Autodesk Inventor part; units mm, degrees
ref_plane "tube_front_XY" through (0, 0, 0) normal (1, 0, 0) x (0, 0, -1)
ref_plane "tube_front_YZ" through (0, 0, 0) normal (0, 0, -1) x (0, 1, 0)
ref_plane "tube_front_ZX" through (0, 0, 0) normal (0, 1, 0) x (1, 0, 0)
sketch "Sketch_1" plane through (0, 0, 0) normal (0, 0, 1) x (1, 0, 0)
  line L0 (414.3629, 0) -> (0, 0)
  arc A0 (-0.6395, 13.2842) -> (-0.6395, 13.1046) centre (-0.5497, 13.1944) ccw
  line L1 (-0.6395, 13.1046) -> (-0.381, 12.846)
  line L2 (-0.381, 12.846) -> (0, 12.846)
  line L3 (0, 12.846) -> (0.762, 13.6081)
  line L4 (0.762, 13.6081) -> (413.6009, 13.6081)
  line L5 (413.6009, 13.6081) -> (414.3629, 12.846)
  line L6 (414.3629, 12.846) -> (414.7439, 12.846)
  line L7 (414.7439, 12.846) -> (415.0024, 13.1046)
  arc A1 (415.0024, 13.1046) -> (415.0024, 13.2842) centre (414.9126, 13.1944) ccw
  line L8 (415.0024, 13.2842) -> (414.3747, 13.9119)
  arc A2 (414.3747, 13.9119) -> (413.8359, 14.1351) centre (413.8359, 13.3731) ccw
  line L9 (413.8359, 14.1351) -> (0.527, 14.1351)
  arc A3 (0.527, 14.1351) -> (-0.0118, 13.9119) centre (0.527, 13.3731) ccw
  line L10 (-0.0118, 13.9119) -> (-0.6395, 13.2842)
revolve "Revolution1" add sketch "Sketch_1" angle 360 about axis through (414.3629, 0, 0) along (1, 0, 0)
ref_plane "tube_front_XY" through (0, 0, 0) normal (1, 0, 0) x (0, 0, -1)
ref_plane "tube_front_YZ" through (0, 0, 0) normal (0, 0, -1) x (0, 1, 0)
ref_plane "tube_front_ZX" through (0, 0, 0) normal (0, 1, 0) x (1, 0, 0)
ref_plane "tube_rear_XY" through (414.3629, 0, 0) normal (1, 0, 0) x (0, 0, -1)
ref_plane "tube_rear_YZ" through (414.3629, 0, 0) normal (0, 0, -1) x (0, 1, 0)
ref_plane "tube_rear_ZX" through (414.3629, 0, 0) normal (0, 1, 0) x (1, 0, 0)
ref_plane "cp1_XY" through (207.1815, 14.1351, 0) normal (1, 0, 0) x (0, 0, -1)
ref_plane "cp1_YZ" through (207.1815, 14.1351, 0) normal (0, 0, -1) x (0, 1, 0)
ref_plane "cp1_ZX" through (207.1815, 14.1351, 0) normal (0, 1, 0) x (1, 0, 0)
ref_plane "cp2_XY" through (207.1815, 0, -14.1351) normal (1, 0, 0) x (0, 0, -1)
ref_plane "cp2_YZ" through (207.1815, 0, -14.1351) normal (0, 0, -1) x (0, 1, 0)
ref_plane "cp2_ZX" through (207.1815, 0, -14.1351) normal (0, 1, 0) x (1, 0, 0)
ref_plane "cp3_XY" through (207.1815, -14.1351, 0) normal (1, 0, 0) x (0, 0, -1)
ref_plane "cp3_YZ" through (207.1815, -14.1351, 0) normal (0, 0, -1) x (0, 1, 0)
ref_plane "cp3_ZX" through (207.1815, -14.1351, 0) normal (0, 1, 0) x (1, 0, 0)
ref_plane "cp4_XY" through (207.1815, 0, 14.1351) normal (1, 0, 0) x (0, 0, -1)
ref_plane "cp4_YZ" through (207.1815, 0, 14.1351) normal (0, 0, -1) x (0, 1, 0)
ref_plane "cp4_ZX" through (207.1815, 0, 14.1351) normal (0, 1, 0) x (1, 0, 0)
properties part number "09R-16.31350" material "Stainless Steel"
Geometry check sheet. Reference: the model listing, model coordinates, mm. Coordinates: 2 decimals unless noted, no trailing zeros. Order: outer loops, then holes, each group sorted by start corner. A loop starts at its lowest first (then second) coordinate and runs counter-clockwise, first axis right, second up.
Item 1: Scan lines: line 1 along Y through (x, z) = (321.5, -1.25); line 2 along Z through (x, y) = (-0.3, 0); line 3 along Z through (x, y) = (414.4, 0). Record each from-to range of solid material in increasing order.
Item 2: Section check A-A (y = 0). Enter the section's corners in (x, z).
Item 3: Mould release check, pull along X, two halves, no side actions. Record for faces 1 (the cylindrical face through (210.07, -10.8, -8.28)), 2 (the cylindrical face through (414.56, -2.78, -12.54)): released by +X, released by -X, zero draft, split by the parting line, or undercut.
Item 4: Section check C-C (x = 251.5). Enter the section's corners in (y, z), plus the area to 3 significant figures.
Item 5: Depth check by flat-ended pin: pin 1 (10 mm diameter, centred on y = 1, z = -7.5, fed in from +X); pin 2 (2 mm diameter, centred on x = 327, y = 10, fed in from +Z); pin 3 (3 mm diameter, centred on x = 300.5, y = 8, fed in from +Z); pin 4 (6 mm diameter, centred on x = 365.5, z = -7.5, fed in from +Y). Enter the tip coordinate at first touch or a pass-through.
Check sheet entries:
1. line 1: y = -14.08 to -13.55, 13.55 to 14.08
1. line 2: z = -13.62 to -12.85, 12.85 to 13.62
1. line 3: z = -13.89 to -12.85, 12.85 to 13.89
2. outline: (-0.64, -13.28) - (-0.01, -13.91) arc R0.76 ccw to (0.53, -14.14) - (413.84, -14.14) arc R0.76 ccw to (414.37, -13.91) - (415, -13.28) arc R0.13 ccw to (415, -13.1) - (414.74, -12.85) - (414.36, -12.85) - (413.6, -13.61) - (0.76, -13.61) - (0, -12.85) - (-0.38, -12.85) - (-0.64, -13.1) arc R0.13 ccw to start; (-0.64, 13.1) - (-0.38, 12.85) - (0, 12.85) - (0.76, 13.61) - (413.6, 13.61) - (414.36, 12.85) - (414.74, 12.85) - (415, 13.1) arc R0.13 ccw to (415, 13.28) - (414.37, 13.91) arc R0.76 ccw to (413.84, 14.14) - (0.53, 14.14) arc R0.76 ccw to (-0.01, 13.91) - (-0.64, 13.28) arc R0.13 ccw to start
3. face 1: undercut
3. face 2: zero draft
4. outline: circle Ø28.27 at (0, 0); hole circle Ø27.22 at (0, 0)
4. area: 45.9 mm2
5. pin 1: passes through
5. pin 2: stops at z = 10.9
5. pin 3: stops at z = 12.55
5. pin 4: stops at y = 13.4
